```python
from build123d import *

# Parameters (mm, degrees)
SKETCH1_W           = 66
SKETCH1_H           = 30
BOSS_EXTRUDE1_DEPTH = 4
FILLET1_R           = 3
SKETCH2_W           = 66
SKETCH2_H           = 30
SKETCH2_W_2         = 58
SKETCH2_H_2         = 22
BOSS_EXTRUDE2_DEPTH = 30
SKETCH3_R           = 10.25
CUT_EXTRUDE1_DEPTH  = 35
SKETCH4_R           = 0.75
CUT_EXTRUDE2_DEPTH  = 35
SKETCH5_W           = 66
SKETCH5_H           = 4
BOSS_EXTRUDE4_DEPTH = 6
SKETCH6_R           = 2.2
CUT_EXTRUDE3_DEPTH  = 6


with BuildPart() as part:
    # Sketch1 → Boss-Extrude1 (new body)
    with BuildSketch(Plane(origin=(0, 0, 0), x_dir=(1, 0, 0), z_dir=(0, 1, 0))):
        with Locations((-33, -15)):
            Rectangle(SKETCH1_W, SKETCH1_H)
    extrude(amount=BOSS_EXTRUDE1_DEPTH)

    # Fillet1
    fillet1_edges = [part.edges().sort_by_distance(p)[0] for p in [
        (-66, 4, 15),
        (-33, 4, 30),
        (0, 4, 15),
        (-33, 4, 0),
    ]]
    fillet(fillet1_edges, radius=FILLET1_R)

    # Sketch2 → Boss-Extrude2 (add)
    with BuildSketch(Plane.XZ):
        with Locations((-33, 15)):
            Rectangle(SKETCH2_W, SKETCH2_H)
        with Locations((-33, 15)):
            Rectangle(SKETCH2_W_2, SKETCH2_H_2, mode=Mode.SUBTRACT)
    extrude(amount=BOSS_EXTRUDE2_DEPTH)

    # Sketch3 → Cut-Extrude1 (cut, through all)
    with BuildSketch(Plane(origin=(0, 4, 0), x_dir=(1, 0, 0), z_dir=(0, 1, 0))):
        with Locations((-33, -15)):
            Circle(SKETCH3_R)
    extrude(amount=-CUT_EXTRUDE1_DEPTH, mode=Mode.SUBTRACT)

    # Sketch4 → Cut-Extrude2 (cut, through all)
    with BuildSketch(Plane(origin=(0, 4, 0), x_dir=(1, 0, 0), z_dir=(0, 1, 0))):
        with Locations((-47.5, -27)):
            Circle(SKETCH4_R)
        with Locations((-18.5, -27)):
            Circle(SKETCH4_R)
    extrude(amount=-CUT_EXTRUDE2_DEPTH, mode=Mode.SUBTRACT)

    # Sketch5 → Boss-Extrude4 (add)
    with BuildSketch(Plane.XZ.offset(30)):
        with Locations((-33, 28)):
            Rectangle(SKETCH5_W, SKETCH5_H)
        with Locations((-33, 2)):
            Rectangle(SKETCH5_W, SKETCH5_H)
    extrude(amount=BOSS_EXTRUDE4_DEPTH)

    # Sketch6 → Cut-Extrude3 (cut)
    with BuildSketch(Plane.XY.offset(30)):
        with Locations((-13, -18)):
            Circle(SKETCH6_R)
    extrude(amount=-CUT_EXTRUDE3_DEPTH, mode=Mode.SUBTRACT)


solid = part.part
```
Verification items for the finished model (mm, model axes). A direction names the side the tool comes from. Coordinates: 2 decimals unless noted, no trailing zeros. Write each loop counter-clockwise with the first axis right and the second up, starting at its lowest first coordinate (ties: lowest second). Pieces come first, ordered by that corner, then holes. Notation, with made-up numbers: M 20.25,7.5 L 36.25,7.5 A31 cw 36.25,43.5 Z; hole C 53.25,10 d7. An arc over 180 degrees is marked long. One line per item, written item: value.
Item 1: Access from +Z, -Z, +X, -X, +Y, -Y to the whole of each face (thin tool, end or side, straight path). Record for faces 4 (the cylindrical face through (-19.095, -12.762, 27.456)), 5 (the cylindrical face through (-65.14, 3.1, 14.79)), 6 (the flat face through (-33, -36, 2)), 7 (the flat face through (-2, -30, 15)), 8 (the flat face through (-33, -18, 26)).
Check sheet entries:
face 4: +Y
face 5: +Z, -Z, -X, +Y
face 6: +Z, -Z, +X, -X, -Y
face 7: +X, -X, -Y
face 8: -Y
Item 2: Section check B-B, the plane y = -7.5. Record the boundary of the cut face in (x, z).
Check sheet entries:
outline: M -66,0 L 0,0 L 0,30 L -66,30 Z; hole M -62,4 L -4,4 L -4,26 L -62,26 Z; hole C -47.5,27 d1.5; hole C -18.5,27 d1.5
Item 3: Section check D-D, the plane x = -5. Record the boundary of the cut face in (y, z).
Check sheet entries:
outline: M -36,0 L 1,0 A3 ccw 4,3 L 4,27 A3 ccw 1,30 L -36,30 L -36,26 L 0,26 L 0,4 L -36,4 Z
Item 4: Mould release check, pull along Z, two halves, no side actions. Record for faces 1 (the flat face through (-4, -15, 15)), 2 (the cylindrical face through (-10.968, -18.843, 28.028)), 3 (the cylindrical face through (-32.54, 3.1, 0.86)): pulls with the +Z half, pulls with the -Z half, needs draft (parallel to the pull), parting line crosses it, or undercut.
Check sheet entries:
face 1: undercut
face 2: needs draft
face 3: pulls with the -Z half
Item 5: Section check A-A, the plane z = 15. Record the boundary of the cut face in (x, y).
Check sheet entries:
outline: M -66,-30 L -62,-30 L -62,0 L -43.25,0 L -43.25,4 L -63,4 A3 ccw -66,1 Z; M -22.75,0 L -4,0 L -4,-30 L 0,-30 L 0,1 A3 ccw -3,4 L -22.75,4 Z
Item 6: Gauge pin test, flat ends, axial feed: pin 1 Ø4.5 at (x, z) = (-64, 14.5) entering from -Y; pin 2 Ø3 at (x, z) = (-14, 7.5) entering from -Y; pin 3 Ø3.5 at (x, y) = (-13, -18) entering from +Z. Record the tip position at first contact, or that the pin passes through.
Check sheet entries:
pin 1: stops at y = -30
pin 2: stops at y = 0
pin 3: stops at z = 4
Item 7: Scan lines: line 1 along X through (y, z) = (-6, 27); line 2 along Z through (x, y) = (-6, -13.5); line 3 along X through (y, z) = (-28, 4.5). Record each from-to range of solid material in increasing order.
Check sheet entries:
line 1: x = -66 to -48.25, -46.75 to -19.25, -17.75 to 0
line 2: z = 0 to 4, 26 to 30
line 3: x = -66 to -62, -4 to 0
Item 8: Section check C-C, the plane x = -13. Record the boundary of the cut face in (y, z).
Check sheet entries:
outline: M -36,0 L 1,0 A3 ccw 4,3 L 4,27 A3 ccw 1,30 L -15.8,30 L -15.8,26 L 0,26 L 0,4 L -36,4 Z; M -36,26 L -20.2,26 L -20.2,30 L -36,30 Z
